from build123d import *

# Parameters (mm, degrees)
F0_W     = 9
F0_H     = 10
F1_DEPTH = 13
F3_DEPTH = 25
F4_W     = 9
F4_H     = 10
F4_H_2   = 15
F5_DEPTH = 3
F6_W     = 9
F6_H     = 10
F7_DEPTH = 8


# Not quite as in the source:
# - a feature names something its author has since deleted; it is built from what else it names


with BuildPart() as f1:
    # F0 (on Top) → F1 (new body)
    with BuildSketch(Plane.XY):
        with Locations((4.5, 5)):
            Rectangle(F0_W, F0_H)
    extrude(amount=F1_DEPTH)

    # F2 (on face) → F3 (cut)
    with BuildSketch(Plane.XZ):
        with BuildLine():
            ThreePointArc((1.5, 13), (4.5, 10), (7.5, 13))
            Line((7.5, 13), (1.5, 13))
        make_face()
    extrude(amount=-F3_DEPTH, mode=Mode.SUBTRACT)

    # F4 (on face) → F5 (join)
    with BuildSketch(Plane(origin=(0, 0, 0), x_dir=(1, 0, 0), z_dir=(0, 0, -1))):
        with Locations((4.5, -5)):
            Rectangle(F4_W, F4_H)
        with Locations((4.5, -17.5)):
            Rectangle(F4_W, F4_H_2)
    extrude(amount=F5_DEPTH)

    # F6 (on face) → F7 (join)
    with BuildSketch(Plane.XY):
        with Locations((4.5, 20)):
            Rectangle(F6_W, F6_H)
    extrude(amount=F7_DEPTH)


solid = f1.part
Part model, mm, in its own coordinate system. A direction names the side the tool comes from. Coordinates: 2 decimals unless noted, no trailing zeros. Write each loop counter-clockwise with the first axis right and the second up, starting at its lowest first coordinate (ties: lowest second). Pieces come first, ordered by that corner, then holes. Notation, with made-up numbers: (19.5, 9) - (74.5, 9) arc R24 cw to (74.5, 47) - close; hole circle Ø8 at (60.25, 34). An arc over 180 degrees is marked (long way). Put each result on its own line as item: value.
1. Flat gauge pins, fed straight in: pin 1 Ø1.5 at (x, z) = (4, 10) entering from +Y; pin 2 Ø4.5 at (x, y) = (4.5, 18.5) entering from +Z; pin 3 Ø1.5 at (y, z) = (17.5, 4) entering from -X. Where does each tip first touch, or does it go through?
Final values:
pin 1: stops at y = 10
pin 2: stops at z = 8
pin 3: stops at x = 0
2. Band-saw the part on A-A (z = 5.25). Write the cut outline in (x, y), then the cut area to 3 significant figures.
Final values:
outline: (0, 0) - (9, 0) - (9, 10) - (0, 10) - close; (0, 15) - (9, 15) - (9, 25) - (0, 25) - close
area: 180 mm²
3. Two-plate mould, pull along Y, no slides. Class faces 1 (the flat face through (4, 15, 4)), 2 (the flat face through (4, 20, 8)), 3 (the flat face through (4, 0, 5)): +Y half, -Y half, draft (parallel to the pull), parting line (faces both ways), or undercut.
Final values:
face 1: undercut
face 2: draft
face 3: -Y half
4. Band-saw the part on D-D (z = 8.25). Write the cut outline in (x, y), then the cut area to 3 significant figures.
Final values:
outline: (0, 0) - (9, 0) - (9, 10) - (0, 10) - close
area: 90.0 mm²
5. Band-saw the part on B-B (x = 4.5). Write the cut outline in (y, z).
Final values:
outline: (0, -3) - (25, -3) - (25, 8) - (15, 8) - (15, 0) - (10, 0) - (10, 10) - (0, 10) - close
6. 3-axis set-ups, long thin cutter, end or side, ignore diameter. For faces 4 (the flat face through (4, 12, -3)), 5 (the flat face through (4, 12, 0)): which of +Z, -Z, +X, -X, +Y, -Y reach the whole face in a straight line?
Final values:
face 4: -Z, +X, -X, +Y, -Y
face 5: +Z, +X, -X
7. Probe line 1 along Z through (x, y) = (4, 13.75); line 2 along Y through (x, z) = (1.25, 3); line 3 along Z through (x, y) = (3, 23.75). List the from-to ranges inside material, lowest first. Write a range as [from, to].
Final values:
line 1: z = [-3, 0]
line 2: y = [0, 10], [15, 25]
line 3: z = [-3, 8]
8. Band-saw the part on C-C (y = 3). Write the cut outline in (x, z), then the cut area to 3 significant figures.
Final values:
outline: (0, -3) - (9, -3) - (9, 13) - (7.5, 13) arc R3 cw to (1.5, 13) - (0, 13) - close
area: 130 mm²
